Source: CAD feature listing. Evaluate the final solid. Frame: model axes, mm. Face numbers are marked on the shaded views. A direction names the side the tool comes from. Coordinates: 2 decimals unless noted, no trailing zeros. Order: outer loops, then holes, each group sorted by start corner. A loop starts at its lowest first (then second) coordinate and runs counter-clockwise, first axis right, second up.
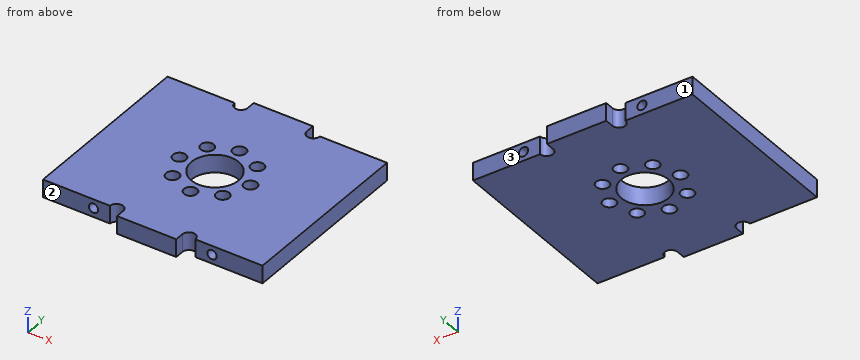
Autodesk Inventor part; units mm, degrees
ref_plane "YZ Plane" through (0, 0, 0) normal (1, 0, 0) x (0, 1, 0)
ref_plane "XZ Plane" through (0, 0, 0) normal (0, 1, 0) x (-1, 0, 0)
ref_plane "XY Plane" through (0, 0, 0) normal (0, 0, 1) x (1, 0, 0)
sketch "スケッチ1" plane through (0, 0, 0) normal (0, 0, 1) x (1, 0, 0)
  circle A0 centre (0, 0) radius 4
  circle A1 centre (0, 0) radius 6 construction
  circle A2 centre (0, 6) radius 1.1
  circle A3 centre (-4.2426, 4.2426) radius 1.1
  circle A4 centre (-6, 0) radius 1.1
  circle A5 centre (-4.2426, -4.2426) radius 1.1
  circle A6 centre (0, -6) radius 1.1
  circle A7 centre (4.2426, -4.2426) radius 1.1
  circle A8 centre (6, 0) radius 1.1
  circle A9 centre (4.2426, 4.2426) radius 1.1
  line L0 (-18.5321, -15.25) -> (18.5321, -15.25)
  line L1 (18.5321, -15.25) -> (18.5321, 15.25)
  line L2 (18.5321, 15.25) -> (-18.5321, 15.25)
  line L3 (-18.5321, 15.25) -> (-18.5321, -15.25)
  line L4 (-18.5321, -15.25) -> (18.5321, 15.25) construction
  line L5 (18.5321, -15.25) -> (-18.5321, 15.25) construction
  circle A10 centre (0, 0) radius 24
  line L6 (18.5321, 0) -> (-18.5321, 0) construction
  line L7 (0, 18.25) -> (0, 0) construction
  line L8 (-5, 15.25) -> (5, 15.25)
  line L9 (5, 15.25) -> (5, 16.75)
  line L10 (5, 16.75) -> (-5, 16.75)
  line L11 (-5, 16.75) -> (-5, 15.25)
  circle A11 centre (-6.1, 15.25) radius 1.1
  circle A12 centre (6.1, 15.25) radius 1.1
  line L12 (-5, -15.25) -> (5, -15.25)
  line L13 (5, -15.25) -> (5, -16.75)
  line L14 (5, -16.75) -> (-5, -16.75)
  line L15 (-5, -16.75) -> (-5, -15.25)
  circle A13 centre (-6.1, -15.25) radius 1.1
  circle A14 centre (6.1, -15.25) radius 1.1
  point P0 (0, 16.75)
  point P1 (0, -18.25)
  point P2 (0, -16.75)
  point P3 (7.2, 15.25)
  point P4 (-7.2, 15.25)
  point P5 (7.2, -15.25)
  point P6 (-7.2, -15.25)
  dimension "d1" = 12
  dimension "d11" = 48
  dimension "d23" = 2.2
  dimension "d24" = 2.2
  dimension "d0" = 8
  dimension "d2" = 2.2
  dimension "d5" = 360
  dimension "d20" = 30.5
  dimension "d21" = 1.5
  dimension "d22" = 10
extrude "押し出し1" add sketch "スケッチ1" along normal blind 3 contours A13 L0 L3 L2 A11 A12 L1 A14 | L0 L13 L14 L15 | L0 A13 | A14 L0 | L2 A11 | A12 L2 | L11 L10 L9 L2 picked at (-6.0558, -14.886) picked at (6.1442, -14.886) picked at (-6.1442, 14.886) picked at (6.0558, 14.886)
extrude "押し出し2" cut sketch "スケッチ1" along normal blind 3 contours L0 A13 | A14 L0 | L2 A11 | A12 L2 picked at (-6.0558, -14.886) picked at (6.1442, -14.886) picked at (-6.1442, 14.886) picked at (6.0558, 14.886)
sketch "スケッチ2" plane through (18.5321, 15.25, 3) normal (0, 1, 0) x (1, 0, 0)
  line L0 (-13.5321, 3) -> (-13.5321, 0)
  line L1 (-23.5321, 3) -> (-23.5321, 0)
  point P0 (-18.5321, 3)
  point P1 (-8.5321, 1.5)
  point P2 (-28.5321, 1.5)
  point P3 (-13.5321, 1.5)
  point P4 (-23.5321, 1.5)
  dimension "d27" = 5
  dimension "d28" = 5
hole "穴1" at (10, 15.25, 1.5) at (-10, 15.25, 1.5) direction (0, -1, 0) diameter 1.567 end through all
properties part number "kosi_sita"
1. Section query A-A, the plane y = 6. Output: boundary loops of the cut face in (x, z).
2. Access query for the marked faces 1, 2 and 3. Directions: +Z, -Z, +X, -X, +Y, -Y. A direction counts if a zero-diameter tool reaches every point of the face in a straight line with its end or side. Return the directions, or none.
3. Material intervals for line 1 along Y through (x, z) = (0, 2); line 2 along X through (y, z) = (-5, 1.4); line 3 along Y through (x, z) = (1, 2.45), sorted ascending.
4. Section query C-C, the plane z = 1.6. Count the separate pieces of the cut face and the enclosed holes in it, plus the area to 3 significant figures.
5. Section query B-B, the plane x = -10. Output: boundary loops of the cut face in (y, z), plus the area to 3 significant figures.
6. Contact query for flat-ended pins moving along their axis: P1, Ø0.8, axis at y = -16.5, z = 1.5, coming from the +X side; P2, Ø1, axis at x = 13, z = 2.5, coming from the -Y side; P3, Ø1.5, axis at x = 15.5, z = 1, coming from the +Y side. Output: stop coordinate, or through.
7. Section query D-D, the plane y = 2. Output: boundary loops of the cut face in (x, z).
Answer key:
1. outline: (-18.53, 0) - (-1.1, 0) - (-1.1, 3) - (-18.53, 3) - close; (1.1, 0) - (18.53, 0) - (18.53, 3) - (1.1, 3) - close; hole circle Ø1.57 at (-10, 1.5); hole circle Ø1.57 at (10, 1.5)
2. face 1: +Z, -Z, -X, +Y
2. face 2: +Z, -Z, -X, -Y
2. face 3: +Z, -Z, +X, +Y
3. line 1: y = -16.75 to -7.1, -4.9 to -4, 4 to 4.9, 7.1 to 16.75
3. line 2: x = -18.53 to -10.78, -9.22 to -5.04, -3.44 to -0.46, 0.46 to 3.44, 5.04 to 9.22, 10.78 to 18.53
3. line 3: y = -16.75 to -6.46, -5.54 to -3.87, 3.87 to 5.54, 6.46 to 16.75
4. separate pieces: 3
4. enclosed holes: 9
4. area: 977 mm2
5. outline: (-15.25, 0) - (15.25, 0) - (15.25, 0.72) - (-15.25, 0.72) - close; (-15.25, 2.28) - (15.25, 2.28) - (15.25, 3) - (-15.25, 3) - close
5. area: 43.7 mm2
6. P1: stops at x = 5
6. P2: stops at y = -15.25
6. P3: stops at y = 15.25
7. outline: (-18.53, 0) - (-3.46, 0) - (-3.46, 3) - (-18.53, 3) - close; (3.46, 0) - (18.53, 0) - (18.53, 3) - (3.46, 3) - close; hole circle Ø1.57 at (-10, 1.5); hole circle Ø1.57 at (10, 1.5)
